Build history of the part. All positions in model axes, mm. A direction names the side the tool comes from. Coordinates: 2 decimals unless noted, no trailing zeros. Write each loop counter-clockwise with the first axis right and the second up, starting at its lowest first coordinate (ties: lowest second). Pieces come first, ordered by that corner, then holes. Notation, with made-up numbers: (-13.75, 21) -> (13.25, 21) arc R21 ccw to (13.25, 47) -> close; hole circle Ø10 at (75.25, 74). An arc over 180 degrees is marked (long way). Write each question's results on one line, items separated by ' | '. Start each with the question number.
Q1. Saw through at C-C on y = 0. Give the cut face in (x, z), and give its area (3 significant figures).
Q2. Two-plate mould, pull along Y, no slides. Class faces 3 (the face through (50.089, 0.209, -26.985)), 4 (the face through (50, -9.525, 124)), 5 (the face through (50, 6.985, 124)): released by +Y, released by -Y, zero draft, split by the parting line, or undercut.
Q3. Drop a flat-ended pin along its axis: pin 1 Ø1 at (x, y) = (20.5, 1) entering from -Z. Give the stop position or say it passes through.
Q4. Tool access for faces 1 (the face through (50.089, 0.154, -24.446)), 2 (the face through (101.6, -8, 134)): list every direction of +Z, -Z, +X, -X, +Y, -Y with a clear straight run to the whole face (end or side of a thin tool).
Q5. Drill centre lines: line 1 (Z direction, x = 76.5, y = 0.75); line 2 (Y direction, x = 56.5, z = 58) (3 decimals); line 3 (Z direction, x = 35.5, y = 4.25). Where is each one in solid material? Low to high.
Q6. Saw through at B-B on z = 237.5. Give the cut face in (x, y) (3 decimals).
Autodesk Inventor part; units mm, degrees
ref_plane "YZ Plane" through (0, 0, 0) normal (1, 0, 0) x (0, 1, 0)
ref_plane "XZ Plane" through (0, 0, 0) normal (0, 1, 0) x (-1, 0, 0)
ref_plane "XY Plane" through (0, 0, 0) normal (0, 0, 1) x (1, 0, 0)
sketch "Sketch1" plane through (0, 0, 0) normal (1, 0, 0) x (0, 1, 0)
  arc A0 (-9.525, -17.4625) -> (9.525, -17.4625) centre (0, -17.4625) ccw
  line L0 (9.525, -17.4625) -> (9.525, 261.9375)
  arc A1 (9.525, 261.9375) -> (-9.525, 261.9375) centre (0, 261.9375) ccw
  line L1 (-9.525, 261.9375) -> (-9.525, -17.4625)
  arc A2 (-6.985, -17.4625) -> (6.985, -17.4625) centre (0, -17.4625) ccw
  arc A3 (6.985, 261.9375) -> (-6.985, 261.9375) centre (0, 261.9375) ccw
  line L2 (6.985, 261.9375) -> (6.985, -17.4625)
  line L3 (-6.985, -17.4625) -> (-6.985, 261.9375)
  point P0 (0, 0)
  dimension "d0" = 9.525
  dimension "d1" = 279.4
  dimension "d2" = 6.985
  dimension "d3" = 6.985
extrude "Extrusion1" add sketch "Sketch1" along normal blind 101.6
sketch "Sketch2" plane through (101.6, 0, 0) normal (1, 0, 0) x (0, 0, -1)
  point P0 (0, 0)
properties part number "BELT"
Returned:
1) outline: (0, -26.99) -> (101.6, -26.99) -> (101.6, -24.45) -> (0, -24.45) -> close; (0, 268.92) -> (101.6, 268.92) -> (101.6, 271.46) -> (0, 271.46) -> close | area: 516 mm2
2) face 3: split by the parting line | face 4: released by -Y | face 5: undercut
3) pin 1: stops at z = -26.97
4) face 1: +X, -X | face 2: +Z, -Z, +X, +Y, -Y
5) line 1: z = -26.96 to -24.41, 268.88 to 271.43 | line 2: y = -9.525 to -6.985, 6.985 to 9.525 | line 3: z = -25.99 to -23.01, 267.48 to 270.46
6) outline: (0, -9.525) -> (101.6, -9.525) -> (101.6, -6.985) -> (0, -6.985) -> close; (0, 6.985) -> (101.6, 6.985) -> (101.6, 9.525) -> (0, 9.525) -> close
